from build123d import *

# Parameters (mm, degrees)
F0_W         = 300
F0_H         = 12
F0_R         = 2
F1_DEPTH     = 15
F3_DEPTH     = 300.001
F4_T4_DEPTH  = 100.0833333333
F4_S5_R      = 2
F4_T6_DEPTH  = 52
F4_T10_DEPTH = 100.1666666667
F4_S11_R     = 2
F4_T12_DEPTH = 52
F4_S13_R     = 2
F4_T14_DEPTH = 52
F4_T18_DEPTH = 100.0833333333
F4_S19_R     = 2
F4_T20_DEPTH = 52
F4_T21_DEPTH = 310.6752080633


# Not quite as in the source:
# - a fillet or chamfer that OpenCascade refuses, or shapes differently, is made with other operations: its cross-section is extruded or revolved along the edge and cut away or added


with BuildPart() as f1:
    # F0 (on Top) → F1 (new body)
    with BuildSketch(Plane.XY):
        Rectangle(F0_W, F0_H)
        with Locations((-50, 0)):
            Circle(F0_R, mode=Mode.SUBTRACT)
        with Locations((50, 0)):
            Circle(F0_R, mode=Mode.SUBTRACT)
    extrude(amount=F1_DEPTH)

    # F2 (on face) → F3 (cut, through all)
    with BuildSketch(Plane.YZ.offset(150)):
        Polygon((6, 15), (-6, 15), (0, 10), align=None)
    extrude(amount=-F3_DEPTH, mode=Mode.SUBTRACT)

    # F4: fillet of radius 1 on 5 edges, made by hand


with BuildPart() as f4_tool2:
    # F4_s3 → F4_t4 (new body)
    with BuildSketch(Plane.YZ.offset(150)):
        with BuildLine():
            ThreePointArc((-0.6401843997, 10.5334869997), (0, 10.3017082793), (0.6401843997, 10.5334869997))
            Line((0.6401843997, 10.5334869997), (0, 10))
            Line((0, 10), (-0.6401843997, 10.5334869997))
        make_face()
    extrude(amount=-F4_T4_DEPTH)

    # F4_s5 → F4_t6 (cut, symmetric)
    with BuildSketch(Plane.XY.offset(10.3)):
        with Locations((50, 0)):
            Circle(F4_S5_R)
    extrude(amount=F4_T6_DEPTH, both=True, mode=Mode.SUBTRACT)


with BuildPart() as f1_1:
    add(f1.part)

    # F4_t1: union F4_tool2
    add(f4_tool2.part)


with BuildPart() as f4_tool8:
    # F4_s9 → F4_t10 (new body)
    with BuildSketch(Plane.YZ.offset(50.0833333333)):
        with BuildLine():
            ThreePointArc((-0.6401843997, 10.5334869997), (0, 10.3017082793), (0.6401843997, 10.5334869997))
            Line((0.6401843997, 10.5334869997), (0, 10))
            Line((0, 10), (-0.6401843997, 10.5334869997))
        make_face()
    extrude(amount=-F4_T10_DEPTH)

    # F4_s11 → F4_t12 (cut, symmetric)
    with BuildSketch(Plane.XY.offset(10.3)):
        with Locations((50, 0)):
            Circle(F4_S11_R)
    extrude(amount=F4_T12_DEPTH, both=True, mode=Mode.SUBTRACT)

    # F4_s13 → F4_t14 (cut, symmetric)
    with BuildSketch(Plane.XY.offset(10.3)):
        with Locations((-50, 0)):
            Circle(F4_S13_R)
    extrude(amount=F4_T14_DEPTH, both=True, mode=Mode.SUBTRACT)


with BuildPart() as f1_2:
    add(f1_1.part)

    # F4_t7: union F4_tool8
    add(f4_tool8.part)


with BuildPart() as f4_tool16:
    # F4_s17 → F4_t18 (new body)
    with BuildSketch(Plane.YZ.offset(-49.9166666667)):
        with BuildLine():
            ThreePointArc((-0.6401843997, 10.5334869997), (0, 10.3017082793), (0.6401843997, 10.5334869997))
            Line((0.6401843997, 10.5334869997), (0, 10))
            Line((0, 10), (-0.6401843997, 10.5334869997))
        make_face()
    extrude(amount=-F4_T18_DEPTH)

    # F4_s19 → F4_t20 (cut, symmetric)
    with BuildSketch(Plane.XY.offset(10.3)):
        with Locations((-50, 0)):
            Circle(F4_S19_R)
    extrude(amount=F4_T20_DEPTH, both=True, mode=Mode.SUBTRACT)


with BuildPart() as f1_3:
    add(f1_2.part)

    # F4_t15: union F4_tool16
    add(f4_tool16.part)

    # F4_s22 → F4_t21 (cut)
    with BuildSketch(Plane.YZ.offset(-155.3376040316)):
        with BuildLine():
            ThreePointArc((-6, 12.8649583873), (-5.4241553962, 13.7705478086), (-4.3598156003, 13.6331796669))
            Line((-4.3598156003, 13.6331796669), (-6, 15))
            Line((-6, 15), (-6, 12.8649583873))
        make_face()
        with BuildLine():
            ThreePointArc((4.3598156003, 13.6331796669), (5.4241553962, 13.7705478086), (6, 12.8649583873))
            Line((6, 12.8649583873), (6, 15))
            Line((6, 15), (4.3598156003, 13.6331796669))
        make_face()
    extrude(amount=F4_T21_DEPTH, mode=Mode.SUBTRACT)


solid = f1_3.part
Here's how the part is built. I have some questions about the finished solid (model axes, mm). Round coordinates to 2 decimals unless told otherwise and drop trailing zeros. Order: outer loops, then holes, each group sorted by start corner. A loop starts at its lowest first (then second) coordinate and runs counter-clockwise, first axis right, second up. Notation, with made-up numbers: (60.5, 1.25) -> (118.5, 1.25) arc R28 cw to (118.5, 39.25) -> close; hole circle Ø9 at (-20.5, -16). An arc over 180 degrees is marked (long way). Use CSV: the item, a comma, the result in double quotes.
1. I need wall thicknesses on line 1 along X through (y, z) = (0, 5); line 2 along Y through (x, z) = (-50, 6); line 3 along X through (y, z) = (-0.5, 2.25). Which ranges of each line are inside material? Lowest first, please.
Recorded:
line 1,"x = -150 to -52, -48 to 48, 52 to 150"
line 2,"y = -6 to -2, 2 to 6"
line 3,"x = -150 to -51.94, -48.06 to 48.06, 51.94 to 150"
2. I want a section at A-A on x = -43.5. List the corners of the cut face in (y, z) for me.
Recorded:
outline,"(-6, 0) -> (6, 0) -> (6, 12.86) arc R1 ccw to (4.36, 13.63) -> (0.64, 10.53) arc R1 cw to (-0.64, 10.53) -> (-4.36, 13.63) arc R1 ccw to (-6, 12.86) -> close"
3. I'm going to push flat-ended pins straight in: P1, Ø3, axis at y = 0.5, z = 10.5, coming from the +X side; P2, Ø3.5, axis at x = 50, y = 0, coming from the -Z side; P3, Ø5, axis at x = 66, y = 1, coming from the +Z side; P4, Ø4, axis at x = -107.5, y = 1, coming from the +Z side. Where does each tip first touch, or does it pass through?
Recorded:
P1,"stops at x = 150"
P2,"passes through"
P3,"stops at z = 12.92"
P4,"stops at z = 12.5"
